```python
from build123d import *

# Parameters (mm, degrees)
BOSS_EXTRUDE1_DEPTH = 2.54
BOSS_EXTRUDE1_TAPER = 15
BOSS_EXTRUDE2_DEPTH = 3.8
FILLET2_R           = 0.1
CHAMFER1_SIZE       = 0.2
BOSS_EXTRUDE3_DEPTH = 3.8
FILLET3_R           = 0.25
FILLET5_R           = 0.5
FILLET6_R           = 0.1
FILLET7_R           = 0.25


with BuildPart() as part:
    # Sketch1 → Boss-Extrude1 (new body)
    with BuildSketch(Plane(origin=(0, 0, 0), x_dir=(1, 0, 0), z_dir=(0, 1, 0))):
        Polygon((-7.62, 5.08), (-7.62, -5.08), (-5.08, -10.16), (5.08, -10.16), (7.62, -5.08), (7.62, 5.08), (5.08, 10.16), (-5.08, 10.16), align=None)
    extrude(amount=BOSS_EXTRUDE1_DEPTH, taper=BOSS_EXTRUDE1_TAPER)

    # Stem → Boss-Extrude2 (add)
    with BuildSketch(Plane.XZ):
        with BuildLine():
            Line((2.499999969, 2.5), (-2.499999969, 2.5))
            ThreePointArc((-2.499999969, 2.5), (-2.85355336, 2.353553391), (-2.999999969, 2))
            Line((-2.999999969, 2), (-2.999999969, -2))
            ThreePointArc((-2.999999969, -2), (-2.85355336, -2.353553391), (-2.499999969, -2.5))
            Line((-2.499999969, -2.5), (2.499999969, -2.5))
            ThreePointArc((2.499999969, -2.5), (2.85355336, -2.353553391), (2.999999969, -2))
            Line((2.999999969, -2), (2.999999969, 2))
            ThreePointArc((2.999999969, 2), (2.85355336, 2.353553391), (2.499999969, 2.5))
        make_face()
        Polygon((-0.5625, 0.6625), (-0.5625, 2.075), (0.5625, 2.075), (0.5625, 0.6625), (2.0625, 0.6625), (2.0625, -0.6625), (0.5625, -0.6625), (0.5625, -2.075), (-0.5625, -2.075), (-0.5625, -0.6625), (-2.0625, -0.6625), (-2.0625, 0.6625), align=None, mode=Mode.SUBTRACT)
    extrude(amount=BOSS_EXTRUDE2_DEPTH)

    # Fillet2
    fillet2_edges = [part.edges().sort_by_distance(p)[0] for p in [
        (2.85355336, -3.8, 2.353553391),
        (0, -3.8, 2.5),
        (2.999999969, -3.8, 0),
        (-2.85355336, -3.8, 2.353553391),
        (-2.999999969, -3.8, 0),
        (-2.85355336, -3.8, -2.353553391),
        (0, -3.8, -2.5),
        (2.85355336, -3.8, -2.353553391),
    ]]
    fillet(fillet2_edges, radius=FILLET2_R)

    # Chamfer1
    chamfer1_edges = [part.edges().sort_by_distance(p)[0] for p in [
        (-2.0625, -3.8, 0),
        (-1.3125, -3.8, 0.6625),
        (-0.5625, -3.8, 1.36875),
        (1.3125, -3.8, 0.6625),
        (-0.5625, -3.8, -1.36875),
        (0, -3.8, 2.075),
        (0.5625, -3.8, 1.36875),
        (2.0625, -3.8, 0),
        (1.3125, -3.8, -0.6625),
        (0.5625, -3.8, -1.36875),
        (-1.3125, -3.8, -0.6625),
    ]]
    chamfer(chamfer1_edges, length=CHAMFER1_SIZE)

    # Sketch3 → Boss-Extrude3 (add)
    with BuildSketch(Plane.XZ):
        Polygon((-7.62, 5.08), (-7.62, -5.08), (-5.08, -10.16), (5.08, -10.16), (7.62, -5.08), (7.62, 5.08), (5.08, 10.16), (-5.08, 10.16), align=None)
        Polygon((-6.35, -4.780193669), (-4.295096834, -8.89), (4.295096834, -8.89), (6.35, -4.780193669), (6.35, 4.780193669), (4.295096834, 8.89), (-4.295096834, 8.89), (-6.35, 4.780193669), align=None, mode=Mode.SUBTRACT)
    extrude(amount=BOSS_EXTRUDE3_DEPTH)

    # Fillet3
    fillet3_edges = [part.edges().sort_by_distance(p)[0] for p in [
        (-6.35, -3.8, 7.62),
        (-7.62, -3.8, 0),
        (-6.35, -3.8, -7.62),
        (0, -3.8, -10.16),
        (6.35, -3.8, -7.62),
        (7.62, -3.8, 0),
        (6.35, -3.8, 7.62),
        (0, -3.8, 10.16),
        (-6.35, -3.8, 0),
        (-5.322548417, -3.8, -6.835096834),
        (0, -3.8, -8.89),
        (5.322548417, -3.8, -6.835096834),
        (6.35, -3.8, 0),
        (5.322548417, -3.8, 6.835096834),
        (0, -3.8, 8.89),
        (-5.322548417, -3.8, 6.835096834),
    ]]
    fillet(fillet3_edges, radius=FILLET3_R)

    # Fillet5
    fillet5_edges = [part.edges().sort_by_distance(p)[0] for p in [
        (-6.35, 0, 0),
        (-5.322548417, 0, -6.835096834),
        (0, 0, -8.89),
        (5.322548417, 0, -6.835096834),
        (6.35, 0, 0),
        (5.322548417, 0, 6.835096834),
        (0, 0, 8.89),
        (-5.322548417, 0, 6.835096834),
        (-2.85355336, 0, 2.353553391),
        (-2.999999969, 0, 0),
        (-2.85355336, 0, -2.353553391),
        (0, 0, -2.5),
        (2.85355336, 0, -2.353553391),
        (2.85355336, 0, 2.353553391),
        (2.999999969, 0, 0),
        (0, 0, 2.5),
    ]]
    fillet(fillet5_edges, radius=FILLET5_R)

    # Fillet6
    fillet6_edges = [part.edges().sort_by_distance(p)[0] for p in [
        (0, 0, 2.075),
        (0.5625, 0, 1.36875),
        (2.0625, 0, 0),
        (1.3125, 0, -0.6625),
        (0.5625, 0, -1.36875),
        (-1.3125, 0, -0.6625),
        (-2.0625, 0, 0),
        (-0.5625, 0, -1.36875),
        (0, 0, -2.075),
        (1.3125, 0, 0.6625),
        (-0.5625, 0, 1.36875),
        (-1.3125, 0, 0.6625),
    ]]
    fillet(fillet6_edges, radius=FILLET6_R)

    # Fillet7
    fillet7_edges = [part.edges().sort_by_distance(p)[0] for p in [
        (-6.939409051, 2.54, 0),
        (-5.799390356, 2.54, 7.199371661),
        (0, 2.54, 9.479409051),
        (5.799390356, 2.54, 7.199371661),
        (6.939409051, 2.54, 0),
        (5.799390356, 2.54, -7.199371661),
        (0, 2.54, -9.479409051),
        (-5.799390356, 2.54, -7.199371661),
    ]]
    fillet(fillet7_edges, radius=FILLET7_R)


solid = part.part
```
Geometry check sheet. Reference: the model listing, model coordinates, mm. A direction names the side the tool comes from. Coordinates: 2 decimals unless noted, no trailing zeros. Answer as a JSON object with one key per item and string values. Group by question number.
Item 1: Scan lines: probe 1 along X at (y, z) = (-2, -1.5); probe 2 along Z at (x, y) = (0.75, -2); probe 3 along Y at (x, z) = (0, -8.25). Record each from-to range of solid material in increasing order.
Item 2: Tool access check on faces 1 (the face through (0, 2.54, 0)), 2 (the face through (5.31, -2, -6.86)). Record the directions out of +Z, -Z, +X, -X, +Y, -Y that give a thin tool (end or side, any length) a straight path to the whole face; none if there is none.
Item 3: Sectioned sample at A-A, the plane y = -2.75. Give the number of separate pieces and of enclosed holes in the cut face, and give its area (3 significant figures).
Item 4: Draft check along Z on faces 3 (the face through (5.21, -0.15, -6.74)), 4 (the face through (1, -2, 0.662)), 5 (the face through (6.265, -3.729, 7.622)), 6 (the face through (-6.268, -3.725, -7.624)). Enter one of: +Z half, -Z half, draft (parallel to the pull), parting line (faces both ways), or undercut.
Resolved:
{
 "1": {"probe 1": "-7.62 to -6.35, -3 to -0.56, 0.56 to 3, 6.35 to 7.62", "probe 2": "-10.16 to -8.89, -2.5 to -0.66, 0.66 to 2.5, 8.89 to 10.16", "probe 3": "0 to 2.54"},
 "2": {"face 1": "+Z, -Z, +X, -X, +Y", "face 2": "-Y"},
 "3": {"separate pieces": "2", "enclosed holes": "2", "area": "96.1 mm^2"},
 "4": {"face 3": "undercut", "face 4": "undercut", "face 5": "+Z half", "face 6": "-Z half"}
}
